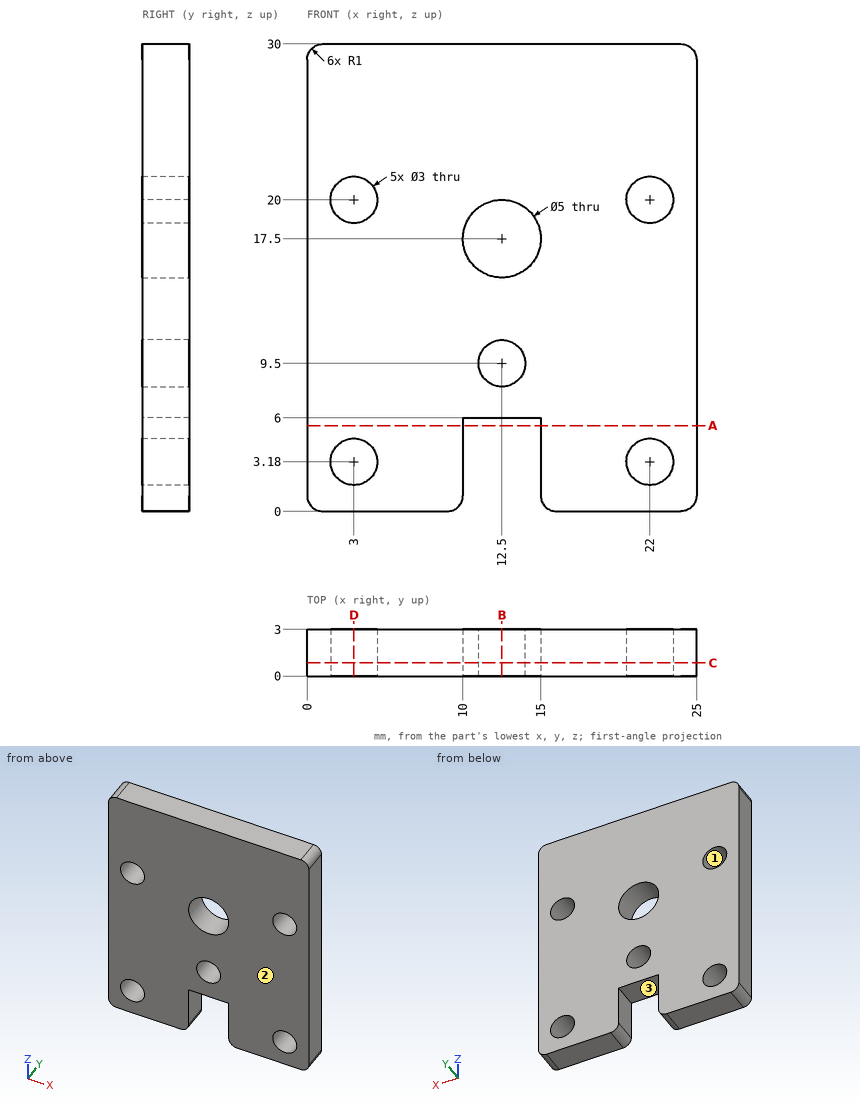
Check sheet for the drawn part. Datum: minimum x, y, z corner. Units: mm. Round coordinates to 2 decimals unless told otherwise and drop trailing zeros. Write each loop counter-clockwise with the first axis right and the second up, starting at its lowest first coordinate (ties: lowest second). Pieces come first, ordered by that corner, then holes. Notation, with made-up numbers: (-0.75, 41) -> (54.25, 41) arc R23 ccw to (54.25, 49) -> close; hole circle Ø6 at (-12.5, 79). An arc over 180 degrees is marked (long way). Write each question's results on one line, items separated by ' | '.
Q1. Sectioned sample at C-C, the plane y = 0.85. Record the boundary of the cut face in (x, z), and give its area (3 significant figures).
Derived:
outline: (0, 1) arc R1 ccw to (1, 0) -> (9, 0) arc R1 ccw to (10, 1) -> (10, 6) -> (15, 6) -> (15, 1) arc R1 ccw to (16, 0) -> (24, 0) arc R1 ccw to (25, 1) -> (25, 29) arc R1 ccw to (24, 30) -> (1, 30) arc R1 ccw to (0, 29) -> close; hole circle Ø3 at (3, 3.18); hole circle Ø3 at (3, 20); hole circle Ø5 at (12.5, 17.5); hole circle Ø3 at (12.5, 9.5); hole circle Ø3 at (22, 3.18); hole circle Ø3 at (22, 20) | area: 664 mm²
Q2. Sectioned sample at D-D, the plane x = 3. Record the boundary of the cut face in (y, z).
Derived:
outline: (0, 0) -> (3, 0) -> (3, 1.68) -> (0, 1.68) -> close; (0, 4.68) -> (3, 4.68) -> (3, 18.5) -> (0, 18.5) -> close; (0, 21.5) -> (3, 21.5) -> (3, 30) -> (0, 30) -> close
Q3. Draft check along Z on the marked faces 1, 2 and 3. Enter one of: released by +Z, released by -Z, zero draft, split by the parting line, or undercut.
Derived:
face 1: undercut | face 2: zero draft | face 3: released by -Z
Q4. Sectioned sample at B-B, the plane x = 12.5. Record the boundary of the cut face in (y, z), and give its area (3 significant figures).
Derived:
outline: (0, 6) -> (3, 6) -> (3, 8) -> (0, 8) -> close; (0, 11) -> (3, 11) -> (3, 15) -> (0, 15) -> close; (0, 20) -> (3, 20) -> (3, 30) -> (0, 30) -> close | area: 48.0 mm²
Q5. Sectioned sample at A-A, the plane z = 5.5. Record the boundary of the cut face in (x, y), and give its area (3 significant figures).
Derived:
outline: (0, 0) -> (10, 0) -> (10, 3) -> (0, 3) -> close; (15, 0) -> (25, 0) -> (25, 3) -> (15, 3) -> close | area: 60.0 mm²
Q6. Thickness scan on probe 1 along X at (y, z) = (1.05, 3.18); probe 2 along X at (y, z) = (1.65, 15.5); probe 3 along Z at (x, y) = (4.25, 2). Record the ranges inside material, lowest first.
Derived:
probe 1: x = 0 to 1.5, 4.5 to 10, 15 to 20.5, 23.5 to 25 | probe 2: x = 0 to 11, 14 to 25 | probe 3: z = 0 to 2.35, 4.01 to 19.17, 20.83 to 30
Q7. Go/stop test with flat-tipped pins: pin 1 Ø3 at (x, z) = (12.5, 17.5) entering from -Y; pin 2 Ø1.5 at (x, y) = (12.5, 1.5) entering from -Z; pin 3 Ø1.5 at (x, y) = (10, 1) entering from -Z. Record where each tip stops, or that it passes through.
Derived:
pin 1: passes through | pin 2: stops at z = 6 | pin 3: stops at z = 0.03
